Build history of the part. All positions in model axes, mm. Face numbers are marked on the shaded views. A direction names the side the tool comes from. Coordinates: 2 decimals unless noted, no trailing zeros. Write each loop counter-clockwise with the first axis right and the second up, starting at its lowest first coordinate (ties: lowest second). Pieces come first, ordered by that corner, then holes. Notation, with made-up numbers: (88, -8.5) -> (94, -8.5) arc R16 cw to (94, 13.5) -> close; hole circle Ø5 at (45.25, -21.75). An arc over 180 degrees is marked (long way). Write each question's results on one line, items separated by ' | '. Start each with the question number.
Q1. Saw through at D-D on z = -35. Give the cut face in (x, y), and give its area (3 significant figures).
Q2. Drill centre lines: line 1 (Y direction, x = 0, z = -32.25); line 2 (X direction, y = 107, z = -35); line 3 (Z direction, x = 5, y = 99). Where is each one in solid material? Low to high.
Q3. Drop flat-ended pins along their axis: pin 1 Ø12 at (x, z) = (30, 10.5) entering from -Y; pin 2 Ø4 at (x, y) = (-27, -3.5) entering from +Z; pin 3 Ø1.5 at (x, y) = (-26, -3.5) entering from -Z. Give the stop position or say it passes through.
Q4. Saw through at A-A on x = 0. Give the cut face in (y, z), and give its area (3 significant figures).
Q5. Saw through at B-B on y = 107.5. Give the cut face in (x, z), and give its area (3 significant figures).
Q6. Tool access for the marked faces 1, 2, 3, 4 and 5: list every direction of +Z, -Z, +X, -X, +Y, -Y with a clear straight run to the whole face (end or side of a thin tool).
Q7. Saw through at C-C on x = -27.5. Give the cut face in (y, z).
from build123d import *

# Parameters (mm, degrees)
SKETCH1_W           = 80
SKETCH1_H           = 100
BOSS_EXTRUDE2_DEPTH = 20
SKETCH2_W           = 25
SKETCH2_H           = 15
BOSS_EXTRUDE3_DEPTH = 100
CUT_EXTRUDE1_REACH  = 150.345
SKETCH3_R           = 5
SKETCH4_W           = 20
SKETCH4_H           = 20
BOSS_EXTRUDE4_DEPTH = 5


with BuildPart() as part:
    # Sketch1 → Boss-Extrude2 (new body)
    with BuildSketch(Plane(origin=(0, 0, 0), x_dir=(1, 0, 0), z_dir=(0, 1, 0))):
        Rectangle(SKETCH1_W, SKETCH1_H)
    extrude(amount=BOSS_EXTRUDE2_DEPTH)

    # Sketch2 → Boss-Extrude3 (add)
    with BuildSketch(Plane(origin=(0, 20, 0), x_dir=(1, 0, 0), z_dir=(0, 1, 0))):
        with Locations((0, 35)):
            Rectangle(SKETCH2_W, SKETCH2_H)
    extrude(amount=BOSS_EXTRUDE3_DEPTH)

    # Sketch3 → Cut-Extrude1 (cut, up to next)
    with BuildSketch(Plane.XY.offset(-27.5), mode=Mode.PRIVATE) as cut_extrude1_sk1:
        with Locations((0, 107.5)):
            Circle(SKETCH3_R)
    cut_extrude1_tool1 = extrude(cut_extrude1_sk1.sketch, amount=-CUT_EXTRUDE1_REACH, mode=Mode.PRIVATE) & part.part
    add(cut_extrude1_tool1.solids().sort_by_distance((0, 107.5, -27.5))[0], mode=Mode.SUBTRACT)

    # Sketch4 → Boss-Extrude4 (add)
    with BuildSketch(Plane.XZ):
        with Locations((-25, 35)):
            Rectangle(SKETCH4_W, SKETCH4_H)
        with Locations((25, 35)):
            Rectangle(SKETCH4_W, SKETCH4_H)
        with Locations((25, -35)):
            Rectangle(SKETCH4_W, SKETCH4_H)
        with Locations((-25, -35)):
            Rectangle(SKETCH4_W, SKETCH4_H)
    extrude(amount=BOSS_EXTRUDE4_DEPTH)


solid = part.part
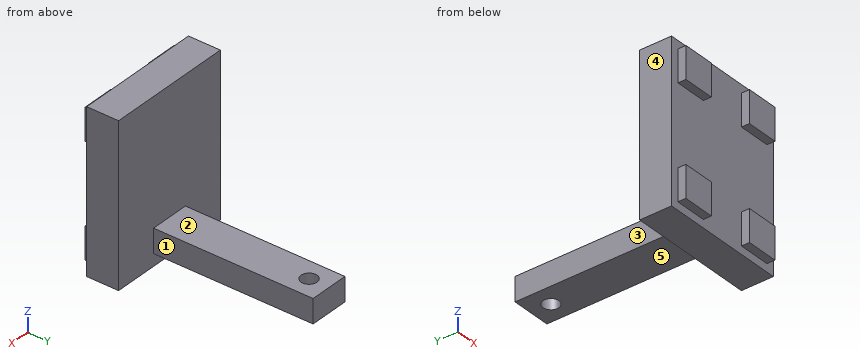
Returned:
1) outline: (-40, 0) -> (-35, 0) -> (-35, -5) -> (-15, -5) -> (-15, 0) -> (15, 0) -> (15, -5) -> (35, -5) -> (35, 0) -> (40, 0) -> (40, 20) -> (12.5, 20) -> (12.5, 120) -> (-12.5, 120) -> (-12.5, 20) -> (-40, 20) -> close; hole circle Ø10 at (0, 107.5) | area: 4,220 mm2
2) line 1: y = 0 to 102.5, 112.5 to 120 | line 2: x = -12.5 to -4.97, 4.97 to 12.5 | line 3: z = -42.5 to -27.5
3) pin 1: stops at y = 0 | pin 2: stops at z = 45 | pin 3: stops at z = -45
4) outline: (0, -50) -> (20, -50) -> (20, -42.5) -> (102.5, -42.5) -> (102.5, -27.5) -> (20, -27.5) -> (20, 50) -> (0, 50) -> close; (112.5, -42.5) -> (120, -42.5) -> (120, -27.5) -> (112.5, -27.5) -> close | area: 3,350 mm2
5) outline: (-12.5, -42.5) -> (-5, -42.5) -> (-5, -27.5) -> (-12.5, -27.5) -> close; (5, -42.5) -> (12.5, -42.5) -> (12.5, -27.5) -> (5, -27.5) -> close | area: 225 mm2
6) face 1: +Z, -Z, +X, +Y | face 2: +Z, +X, -X, +Y | face 3: +Z, -Z, -X, +Y | face 4: +Z, -Z, -X, +Y, -Y | face 5: -Z, +X, -X, +Y
7) outline: (-5, -45) -> (0, -45) -> (0, -50) -> (20, -50) -> (20, 50) -> (0, 50) -> (0, 45) -> (-5, 45) -> (-5, 25) -> (0, 25) -> (0, -25) -> (-5, -25) -> close
